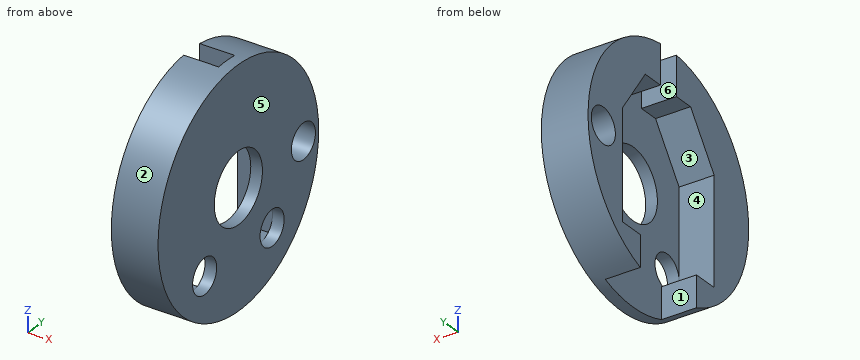
Autodesk Inventor part; units mm, degrees
ref_plane "YZ Plane" through (0, 0, 0) normal (1, 0, 0) x (0, 1, 0)
ref_plane "XZ Plane" through (0, 0, 0) normal (0, 1, 0) x (-1, 0, 0)
ref_plane "XY Plane" through (0, 0, 0) normal (0, 0, 1) x (1, 0, 0)
sketch "Sketch1" plane through (0, 0, 0) normal (1, 0, 0) x (0, 1, 0)
  circle A0 centre (0, 0) radius 10
  line L0 (10, 0) -> (8.1, 0)
  circle A1 centre (8.1, 0) radius 1.5
  circle A2 centre (0, 0) radius 3
  dimension "d0" = 20
  dimension "d1" = 1.9
  dimension "d2" = 3
  dimension "d3" = 6
extrude "Extrusion1" add sketch "Sketch1" along normal blind 1
sketch "Sketch2" plane through (0, 0, 0) normal (-1, 0, 0) x (0, 0, 1)
  line L0 (0, 5.5) -> (-6.5, 5.5)
  line L1 (0, 5.5) -> (2.5, 5.5)
  line L2 (6.0478, 3.0122) -> (6.0478, -2.8019)
  line L3 (-6.5, -5.5) -> (-6.5, 5.5)
  line L4 (5.5, 5.498) -> (2.5, 5.5)
  line L5 (2.5, 5.5) -> (6.0478, 3.0122)
  line L6 (5.2, -5.498) -> (2.2, -5.5)
  line L7 (2.2, -5.5) -> (6.0478, -2.8019)
  line L8 (2.2, -5.5) -> (-6.5, -5.5)
  line L9 (2.5631, 5.7) -> (6.585, 2.8798)
  line L10 (6.585, 2.8798) -> (6.585, -2.7667)
  line L11 (6.585, -2.7667) -> (2.4018, -5.7)
  line L12 (2.5631, 5.7) -> (0, 5.7)
  line L13 (0, 5.7) -> (-6.7, 5.7)
  line L14 (-6.7, 5.7) -> (-6.7, -5.7)
  line L15 (-6.7, -5.7) -> (2.4018, -5.7)
  circle A0 centre (0, 0) radius 10
  circle A1 centre (0, 0) radius 10
  line L16 (10, 0) -> (10, 1)
  line L17 (10, 1) -> (6.585, 1)
  line L18 (10, 0) -> (10, -1)
  line L19 (10, 0) -> (11, 0) construction
  line L20 (10, -1) -> (6.585, -1)
  line L21 (-10, 0) -> (-10, 3.5)
  line L22 (-10, 3.5) -> (-6.7, 3.5)
  line L23 (-10, 0) -> (-10, -3.5)
  line L24 (-10, -3.5) -> (-6.7, -3.5)
  circle A2 centre (0, 8.1) radius 1.5
  circle A3 centre (0, 8.1) radius 1.5
  point P0 (-9.3675, -3.5)
  point P1 (9.9499, -1)
  point P2 (9.9499, 1)
  point P3 (-9.3675, 3.5)
  dimension "d6" = 5.5
  dimension "d7" = 6.5
  dimension "d8" = 5.5
  dimension "d9" = 11
  dimension "d10" = 3
  dimension "d11" = 35
  dimension "d12" = 3
  dimension "d13" = 35
  dimension "d14" = 0.2
  dimension "d15" = 0.2
  dimension "d18" = 1
  dimension "d19" = 1
  dimension "d20" = 270
  dimension "d21" = 3.5
  dimension "d22" = 3.5
extrude "Extrusion2" add sketch "Sketch2" along normal blind 3 contours L9 L12 L13 L14 L22 A0 L17 L10 | L11 L10 L20 A0 L24 L14 L15
sketch "Sketch3" plane through (0, 0, 0) normal (-1, 0, 0) x (0, 0, 1)
  circle A0 centre (-5.2, 4.2) radius 1.5
  circle A1 centre (-5.2, -4.2) radius 1.5
  line L0 (-6.7, 5.7) -> (2.5631, 5.7)
  line L1 (-6.7, 3.5) -> (-6.7, 5.7)
  line L2 (-6.7, -5.7) -> (-6.7, -3.5)
  line L3 (2.4018, -5.7) -> (-6.7, -5.7)
  point P0 (0, 0)
  dimension "d23" = 3
  dimension "d24" = 3
extrude "Extrusion3" cut sketch "Sketch3" against normal blind 10 contours A0 | A1
properties part number "potentiometer_holder"
Input: part model. Units: mm. Frame: model coordinates. Face numbers are marked on the shaded views. A direction names the side the tool comes from. Coordinates: 2 decimals unless noted, no trailing zeros. Loops run counter-clockwise (first coordinate to the right, second up) from the corner with the lowest first, then second, coordinate; pieces in that order, holes last.
Q1. Section B-B, the plane x = -0.4. Return the cut outline in (y, z) (1 decimal), and give its area (3 significant figures).
Results are:
outline: (-5.7, -6.7) - (-5.7, 2.4) - (-2.8, 6.6) - (-1, 6.6) - (-1, 9.9) arc R10 ccw to (-3.5, -9.4) - (-3.5, -6.7) - close; (1, 6.6) - (2.9, 6.6) - (5.7, 2.6) - (5.7, -6.7) - (3.5, -6.7) - (3.5, -9.4) arc R10 ccw to (1, 9.9) - close; hole circle Ø3 at (8.1, 0)
area: 139 mm2
Q2. Set-up query: the marked faces 4, 5 and 6. Return all of +Z, -Z, +X, -X, +Y, -Y with unobstructed straight access to the full face (end or side cutting, diameter ignored); none if empty.
Results are:
face 4: -X
face 5: +Z, -Z, +X, +Y, -Y
face 6: +Z, -Z, -X
Q3. Section A-A, the plane y = 0. Return the cut outline in (x, z).
Results are:
outline: (0, -10) - (1, -10) - (1, -3) - (0, -3) - close; (0, 3) - (1, 3) - (1, 10) - (0, 10) - close
Q4. Mould query, pull axis Z, two halves, no side actions, for the marked faces 1, 2 and 3. Classes: +Z half, -Z half, draft (parallel to the pull), parting line (faces both ways), or undercut.
Results are:
face 1: draft
face 2: parting line
face 3: undercut
Q5. Contact query for flat-ended pins moving along their axis: pin 1 (0.6 mm diameter, centred on x = -1.5, y = 2, fed in from -Z) (3 decimals); pin 2 (0.9 mm diameter, centred on x = -1, z = -2.5, fed in from +Y); pin 3 (2 mm diameter, centred on x = -1.5, z = -2, fed in from +Y). Output: stop coordinate, or through.
Results are:
pin 1: stops at z = 6.585
pin 2: stops at y = 9.79
pin 3: stops at y = 9.95
Q6. Section D-D, the plane x = 0.65. Return the cut outline in (y, z).
Results are:
outline: circle Ø20 at (0, 0); hole circle Ø3 at (-4.2, -5.2); hole circle Ø6 at (0, 0); hole circle Ø3 at (4.2, -5.2); hole circle Ø3 at (8.1, 0)
Q7. Line query: line 1 along Y through (x, z) = (-0.9, 0); line 2 along Z through (x, y) = (0.7, 0); line 3 along Y through (x, z) = (0.65, -5.2). Output: solid intervals per line, ascending.
Results are:
line 1: y = -10 to -5.7, 5.7 to 6.6, 9.6 to 10
line 2: z = -10 to -3, 3 to 10
line 3: y = -8.54 to -5.7, -2.7 to 2.7, 5.7 to 8.54
Q8. Section C-C, the plane z = -1. Return the cut outline in (x, y).
Results are:
outline: (-3, -9.95) - (1, -9.95) - (1, -2.83) - (0, -2.83) - (0, -5.7) - (-3, -5.7) - close; (-3, 5.7) - (0, 5.7) - (0, 2.83) - (1, 2.83) - (1, 6.98) - (-3, 6.98) - close; (-3, 9.22) - (1, 9.22) - (1, 9.95) - (-3, 9.95) - close
